Autodesk Inventor part; units mm, degrees
ref_plane "WorkPlane1" through (0, 0, 0) normal (0, 0, 1) x (1, 0, 0)
ref_plane "MSC_PF1" through (0, 0, 0) normal (1, 0, 0) x (0, 1, 0)
ref_plane "MSC_PT1" through (0, 0, 0) normal (0, 0, -1) x (-1, 0, 0)
ref_plane "WorkPlane1" through (0, 0, 0) normal (0, 0, 1) x (1, 0, 0)
sketch "Sketch1" plane through (0, 0, 0) normal (0, 0, 1) x (1, 0, 0)
  point P0 (0, 0)
sketch "Sketch2" plane through (0, 0, 0) normal (0, 0, 1) x (1, 0, 0)
  line L0 (-12, 6.9284) -> (-12, -6.9284)
  line L1 (0, 13.8562) -> (-12, 6.9284)
  line L2 (12, 6.9284) -> (0, 13.8562)
  line L3 (12, -6.9284) -> (12, 6.9284)
  line L4 (0, -13.8562) -> (12, -6.9284)
  line L5 (-12, -6.9284) -> (0, -13.8562)
  circle A0 centre (0, 0) radius 12 construction
  dimension "d1" = 24
  dimension "d29" = 0
  dimension "d30" = 0
extrude "Extrusion1" add sketch "Sketch2" along normal blind 10
sketch "Sketch3" plane through (0, 0, 0) normal (1, 0, 0) x (0, 1, 0)
  line L0 (12, 10) -> (13.9562, 10)
  line L1 (13.9562, 8.8706) -> (12, 10)
  line L2 (13.9562, 10) -> (13.9562, 8.8706)
  line L3 (0, -2) -> (0, 12)
  line L4 (13.8562, 0) -> (13.8562, 10)
  dimension "d25" = 0.1
  dimension "d26" = 0
  dimension "d27" = 60
  dimension "d28" = 12
revolve "Revolution1" cut sketch "Sketch3" angle 360 about axis through (0, 0, -10) along (0, 0, 1)
sketch "Sketch4" plane through (0, 0, 0) normal (1, 0, 0) x (0, 1, 0)
  line L0 (0, -65) -> (0, 0)
  line L1 (-8, -65) -> (0, -65)
  line L2 (-8, 0) -> (-8, -65)
  line L3 (0, 0) -> (-8, 0)
  line L4 (0, -65) -> (0, 0)
  line L5 (-9.6, 0) -> (1.6, 0)
  line L6 (0, -78) -> (0, 13)
  dimension "d18" = 8
  dimension "d20" = 65
  dimension "d33" = 0
  dimension "d34" = 0
revolve "Revolution2" add sketch "Sketch4" angle 360 about axis through (0, 0, -65) along (0, 0, -1)
chamfer "Chamfer1" distance 1 angle 45 1 edges at (0, 8, -65)
fillet "Fillet1" radius 0.6 1 edges at (0, 8, 0)
thread "Thread1"
ref_plane "MSC_PF1" through (0, 0, 0) normal (1, 0, 0) x (0, 1, 0)
ref_plane "MSC_PT1" through (0, 0, 0) normal (0, 0, -1) x (-1, 0, 0)
equation "\"d22\" = 0.5 * PTC"
equation "\"d23\" = 0.5 * PTC"
equation "\"d24\" = r"
equation "\"d1\" = ParS"
equation "\"d6\" = ParK"
equation "\"d28\" = 0.5 * ParS"
equation "\"d18\" = 0.5 * NND"
equation "\"d20\" = NLG"
equation "\"NND\" = 16"
equation "\"NLG\" = 65"
equation "\"PTC\" = 2"
equation "\"ParK\" = 10"
equation "\"ParS\" = 24"
equation "\"msp_es\" = 0.577367 * ParS"
equation "\"r\" = 0.6"
equation "\"THREADDIA\" = NND"
properties part number "ISO 4016 - M16 x 65" material "Steel"
Read the model definition and answer for the solid it produces. Units are mm, in the model's axes. A direction names the side the tool comes from. Give positions to 0.01 mm unless a question says otherwise; leave off trailing zeros. Order: outer loops, then holes, each group sorted by start corner. A loop starts at its lowest first (then second) coordinate and runs counter-clockwise, first axis right, second up. Notation, with made-up numbers: (16, 35.5) -> (43, 35.5) arc R28 ccw to (43, 66.5) -> close; hole circle Ø3 at (-33, -26). An arc over 180 degrees is marked (long way). One line per item, written item: value. Start each with the question number.
(1) Flat-ended cylindrical pins translate along their axes: P1, Ø4, axis at x = -6.5, z = -25, coming from the +Y side; P2, Ø8, axis at y = -0.5, z = -40, coming from the -X side; P3, Ø12, axis at y = 9.5, z = -24, coming from the -X side. Find the tip coordinate at first contact, or state that the pin passes through.
(2) A tool of negligible diameter and unlimited length cuts with its end or side. For faces 1 (the flat face through (0, 0, 10)), 2 (the flat face through (0, -9, 0)), from which of +Z, -Z, +X, -X, +Y, -Y can it reach the whole face along a straight path? Write none if from no direction.
(3) The part is cut by section A-A (z = -48.5). Determine the outline of the cut face in (x, y), and give its area (3 significant figures).
(4) Straight lines are drawn through the part: L1, parallel to Y at x = 0.5, z = -6.5; L2, parallel to Z at x = 7.75, y = 3.5. For each, find the intervals that lie inside material, in ascending order.
Taken from the geometry:
1. P1: y = 6.61
1. P2: x = -8
1. P3: x = -7.19
2. face 1: +Z, +X, -X, +Y, -Y
2. face 2: -Z
3. outline: circle Ø16 at (0, 0)
3. area: 201 mm^2
4. L1: -7.98 to 7.98
4. L2: -0.01 to 10
